Check sheet for the modelled part. Datum: model origin and axes. Units: mm. A direction names the side the tool comes from. Coordinates: 2 decimals unless noted, no trailing zeros. Loops run counter-clockwise (first coordinate to the right, second up) from the corner with the lowest first, then second, coordinate; pieces in that order, holes last. Notation, with made-up numbers: (-27.5, 73.25) - (20.5, 73.25) arc R14 ccw to (20.5, 87.25) - close; hole circle Ø8 at (-33.75, -22.5). An arc over 180 degrees is marked (long way). Answer as a JSON object with one key per item and string values. Group by question number.
from build123d import *

# Parameters (mm, degrees)
F0_W     = 78
F0_H     = 60
F1_DEPTH = 21.5
F2_W     = 76
F2_H     = 58
F3_DEPTH = 20
F5_DEPTH = 60.001
F6_W     = 0.5
F6_H     = 1.5
F7_DEPTH = 4
F8_R     = 1.5
F9_DEPTH = 25


with BuildPart() as f1:
    # F0 (on Top) → F1 (new body)
    with BuildSketch(Plane.XY):
        with Locations((39, -30)):
            Rectangle(F0_W, F0_H)
    extrude(amount=F1_DEPTH)

    # F2 (on face) → F3 (cut)
    with BuildSketch(Plane.XY.offset(21.5)):
        with Locations((39, -30)):
            Rectangle(F2_W, F2_H)
    extrude(amount=-F3_DEPTH, mode=Mode.SUBTRACT)

    # F4 (on face) → F5 (cut, through all)
    with BuildSketch(Plane.XZ.offset(60)):
        Polygon((27.707402, 9.04668), (39, 9.04668), (50.292598, 9.04668), (53.762321, 12.020729), (63.345369, 12.020729), (68.136893, 15.65568), (76.232917, 15.65568), (76.232917, 21.5), (1.767083, 21.5), (1.767083, 15.65568), (9.863107, 15.65568), (14.654631, 12.020729), (24.237679, 12.020729), align=None)
    extrude(amount=-F5_DEPTH, mode=Mode.SUBTRACT)

    # F6 (on face) → F7 (join)
    with BuildSketch(Plane(origin=(0, 0, 0), x_dir=(1, 0, 0), z_dir=(0, 0, -1))):
        with Locations((75, 10.5)):
            Rectangle(F6_W, F6_H)
        with Locations((75, 30)):
            Rectangle(F6_W, F6_H)
        with Locations((75, 49.5)):
            Rectangle(F6_W, F6_H)
        with Locations((3, 10.5)):
            Rectangle(F6_W, F6_H)
        with Locations((3, 49.5)):
            Rectangle(F6_W, F6_H)
        with Locations((3, 30)):
            Rectangle(F6_W, F6_H)
    extrude(amount=F7_DEPTH)

    # F8 (on face) → F9 (cut)
    with BuildSketch(Plane(origin=(0, 0, 0), x_dir=(1, 0, 0), z_dir=(0, 0, -1))):
        with BuildLine():
            ThreePointArc((65.5, 10.5), (67, 9), (68.5, 10.5))
            Line((68.5, 10.5), (65.5, 10.5))
        make_face()
        with BuildLine():
            Line((65.5, 10.5), (68.5, 10.5))
            ThreePointArc((68.5, 10.5), (67, 12), (65.5, 10.5))
        make_face()
        with BuildLine():
            ThreePointArc((9.5, 10.5), (11, 9), (12.5, 10.5))
            Line((12.5, 10.5), (9.5, 10.5))
        make_face()
        with BuildLine():
            Line((9.5, 10.5), (12.5, 10.5))
            ThreePointArc((12.5, 10.5), (11, 12), (9.5, 10.5))
        make_face()
        with BuildLine():
            ThreePointArc((65.5, 30), (67, 28.5), (68.5, 30))
            Line((68.5, 30), (65.5, 30))
        make_face()
        with BuildLine():
            Line((65.5, 30), (68.5, 30))
            ThreePointArc((68.5, 30), (67, 31.5), (65.5, 30))
        make_face()
        with BuildLine():
            ThreePointArc((9.5, 30), (11, 28.5), (12.5, 30))
            Line((12.5, 30), (9.5, 30))
        make_face()
        with BuildLine():
            Line((9.5, 30), (12.5, 30))
            ThreePointArc((12.5, 30), (11, 31.5), (9.5, 30))
        make_face()
        with Locations((67, 49.5)):
            Circle(F8_R)
        with Locations((11, 49.5)):
            Circle(F8_R)
    extrude(amount=-F9_DEPTH, mode=Mode.SUBTRACT)


solid = f1.part
1. Gauge pin test, flat ends, axial feed: pin 1 (10 mm diameter, centred on x = 15.5, y = -10.5, fed in from +Z); pin 2 (5 mm diameter, centred on x = 37.5, y = -26.5, fed in from -Z); pin 3 (1.2 mm diameter, centred on y = -50, z = -1, fed in from -X). Record the tip position at first contact, or that the pin passes through.
2. Sectioned sample at C-C on x = 11. Record the cut outline in (y, z), plus the area to 3 significant figures.
3. Material ranges on line 1 (X direction, y = -30, z = 1.1); line 2 (Y direction, x = 11, z = 0.9); line 3 (X direction, y = -4, z = 16.5), recorded low to high.
4. Release check for a two-part mould opening along X. For faces 4 (the face through (78, -30, 11)), 5 (the face through (38, 0, 6)), 6 (the face through (25.948, -59.507, 10.555)), 7 (the face through (0, -30, 11)) record: released by +X, released by -X, zero draft, split by the parting line, or undercut.
5. Sectioned sample at A-A on x = 46. Record the cut outline in (y, z), plus the area to 3 significant figures.
6. Access from +Z, -Z, +X, -X, +Y, -Y to the whole of each face (thin tool, end or side, straight path). Record for faces 1 (the face through (68.43, -10.95, 0.74)), 2 (the face through (1, -30, 12)), 3 (the face through (12.23, -59.51, 13.86)).
7. Sectioned sample at B-B on y = -8. Record the cut outline in (x, z).
Answers follow:
{
 "1": {"pin 1": "stops at z = 1.5", "pin 2": "stops at z = 0", "pin 3": "stops at x = 2.75"},
 "2": {"outline": "(-60, 0) - (-51, 0) - (-51, 1.5) - (-59, 1.5) - (-59, 14.79) - (-60, 14.79) - close; (-48, 0) - (-31.5, 0) - (-31.5, 1.5) - (-48, 1.5) - close; (-28.5, 0) - (-12, 0) - (-12, 1.5) - (-28.5, 1.5) - close; (-9, 0) - (0, 0) - (0, 14.79) - (-1, 14.79) - (-1, 1.5) - (-9, 1.5) - close", "area": "103 mm^2"},
 "3": {"line 1": "x = 0 to 9.5, 12.5 to 65.5, 68.5 to 78", "line 2": "y = -60 to -51, -48 to -31.5, -28.5 to -12, -9 to 0", "line 3": "x = 0 to 1, 77 to 78"},
 "4": {"face 4": "released by +X", "face 5": "zero draft", "face 6": "undercut", "face 7": "released by -X"},
 "5": {"outline": "(-60, 0) - (0, 0) - (0, 9.05) - (-1, 9.05) - (-1, 1.5) - (-59, 1.5) - (-59, 9.05) - (-60, 9.05) - close", "area": "105 mm^2"},
 "6": {"face 1": "+Z, -Z", "face 2": "+Z", "face 3": "+Z, +Y, -Y"},
 "7": {"outline": "(0, 0) - (78, 0) - (78, 21.5) - (77, 21.5) - (77, 1.5) - (1, 1.5) - (1, 21.5) - (0, 21.5) - close"}
}
